For this review, take the finished solid that the model builds, in its own axes (mm). Face numbers are marked on the shaded views. A direction names the side the tool comes from. Coordinates: 2 decimals unless noted, no trailing zeros. Loops run counter-clockwise (first coordinate to the right, second up) from the corner with the lowest first, then second, coordinate; pieces in that order, holes last.
1. Take a section at C-C, the plane x = 1.2. State the section outline as (y, z) points, then the cut area to 3 significant figures.
2. Take a section at D-D, the plane z = 1.5. State the section outline as (x, y) points.
3. Clearance check with flat-ended pins moving along their axes: P1, Ø1, axis at x = 1.5, y = -0.5, coming from the +Z side; P2, Ø1, axis at x = -1, y = 4.5, coming from the +Z side; P3, Ø1, axis at y = 1.5, z = 1.5, coming from the -X side. State where each tip first meets the part, or that it passes through.
4. Take a section at A-A, the plane y = -0.5. State the section outline as (x, z) points (3 decimals), then the cut area to 3 significant figures.
5. Machinability: for the marked faces 1 and 2, which of the approach directions +Z, -Z, +X, -X, +Y, -Y give a long, thin tool a straight path to every point of the face, cutting with its end or side? Answer none if there is none.
6. To check wall thickness, follow probe 1 along Y at (x, z) = (0.4, -0.55); probe 2 along Z at (x, y) = (0.95, 4.5); probe 3 along Z at (x, y) = (1.35, 0.25). State the ranges of each line that lie inside material, in increasing order.
7. Take a section at B-B, the plane z = 0.1. State the section outline as (x, y) points (3 decimals).
8. Mouldability with a two-part tool opening along X and no side actions: class the marked faces 3, 4 and 5 as pulls with the +X half, pulls with the -X half, needs draft (parallel to the pull), parting line crosses it, or undercut.
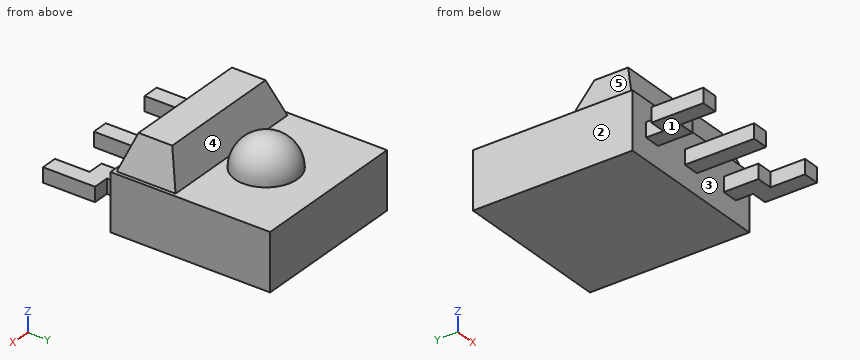
```python
from build123d import *

# Parameters (mm, degrees)
BOSS_EXTRUDE1_DEPTH   = 0.21
SKETCH1_W             = 0.47
SKETCH1_H             = 2
BOSS_EXTRUDE1_2_DEPTH = 0.21
BOSS_EXTRUDE1_3_DEPTH = 0.21
SKETCH2_W             = 4.6
SKETCH2_H             = 1.64
BOSS_EXTRUDE2_DEPTH   = 4.6
REVOLVE1_ANGLE        = 180
SKETCH4_W             = 4.4
SKETCH4_H             = 1.7
BOSS_EXTRUDE3_DEPTH   = 1
CHAMFER1_SIZE         = 1
CHAMFER1_SIZE_2       = 0.363970234


with BuildPart() as part:
    # Sketch1 → Boss-Extrude1 (new, symmetric)
    with BuildSketch(Plane.XY):
        Polygon((-1.295, 1), (-1.295, 0), (-1.765, 0), (-1.765, -1), (-2.235, -1), (-2.235, 0.5), (-1.765, 0.5), (-1.765, 1), align=None)
    extrude(amount=BOSS_EXTRUDE1_DEPTH, both=True)



with BuildPart() as body_2:
    # Sketch1 → Boss-Extrude1 2 (new, symmetric)
    with BuildSketch(Plane.XY):
        Rectangle(SKETCH1_W, SKETCH1_H)
    extrude(amount=BOSS_EXTRUDE1_2_DEPTH, both=True)


with BuildPart() as body_3:
    # Sketch1 → Boss-Extrude1 3 (new, symmetric)
    with BuildSketch(Plane.XY):
        Polygon((1.765, 1), (1.295, 1), (1.295, 0), (1.765, 0), (1.765, -1), (2.235, -1), (2.235, 0.5), (1.765, 0.5), align=None)
    extrude(amount=BOSS_EXTRUDE1_3_DEPTH, both=True)


with BuildPart() as part_1:
    add(part.part)

    add(body_2.part)  # Boss-Extrude2 merges body 2

    add(body_3.part)  # Boss-Extrude2 merges body 3
    # Sketch2 → Boss-Extrude2 (add)
    with BuildSketch(Plane(origin=(0, 1, 0), x_dir=(1, 0, 0), z_dir=(0, 1, 0))):
        Rectangle(SKETCH2_W, SKETCH2_H)
    extrude(amount=BOSS_EXTRUDE2_DEPTH)

    # Sketch3 → Revolve1 (revolve)
    with BuildSketch(Plane.XY.offset(0.82)):
        with BuildLine():
            Line((0, 4.7), (0, 2.9))
            ThreePointArc((0, 2.9), (0.9, 3.8), (0, 4.7))
        make_face()
    revolve(axis=Axis((0, 4.7, 0.82), (0, -1, 0)), revolution_arc=REVOLVE1_ANGLE)

    # Sketch4 → Boss-Extrude3 (add)
    with BuildSketch(Plane.XY.offset(0.82)):
        with Locations((0, 1.95)):
            Rectangle(SKETCH4_W, SKETCH4_H)
    extrude(amount=BOSS_EXTRUDE3_DEPTH)

    # Chamfer1
    # the kernel refuses this chamfer: 1, 0.363970234 mm, written as the material it takes off along each edge
    with BuildSketch(Plane(origin=(4.794194733, 1.1, 1.82), x_dir=(0, -0.013184058198646006, -0.9999130865277315), z_dir=(-1, 0, 0))) as chamfer1_piece_1_section:
        Polygon((CHAMFER1_SIZE * 0.999913086528, -CHAMFER1_SIZE * 0.0131840581986), (-CHAMFER1_SIZE_2 * 0.0131840582083, -CHAMFER1_SIZE_2 * 0.999913087259), (0, 0), align=None)
    chamfer1_piece_1 = extrude(amount=9.588389465, mode=Mode.PRIVATE)
    chamfer1_piece_1 = split(chamfer1_piece_1, bisect_by=Plane(origin=(0, 1.212526608, 0.82), z_dir=(0, 0, 1)), keep=Keep.TOP, mode=Mode.PRIVATE)
    add(chamfer1_piece_1, mode=Mode.SUBTRACT)
    with BuildSketch(Plane(origin=(-2.2, -1.494194733, 1.82), x_dir=(-0.013184058198646006, 0, -0.9999130865277315), z_dir=(0, 1, 0))) as chamfer1_piece_2_section:
        Polygon((CHAMFER1_SIZE * 0.999913086528, -CHAMFER1_SIZE * 0.0131840581986), (-CHAMFER1_SIZE_2 * 0.0131840582083, -CHAMFER1_SIZE_2 * 0.999913087259), (0, 0), align=None)
    chamfer1_piece_2 = extrude(amount=6.888389465, mode=Mode.PRIVATE)
    chamfer1_piece_2 = split(chamfer1_piece_2, bisect_by=Plane(origin=(-2.087473392, 1.95, 0.82), z_dir=(0, 0, 1)), keep=Keep.TOP, mode=Mode.PRIVATE)
    add(chamfer1_piece_2, mode=Mode.SUBTRACT)
    with BuildSketch(Plane(origin=(2.2, 5.394194733, 1.82), x_dir=(0.013184058198646006, 0, -0.9999130865277315), z_dir=(0, -1, 0))) as chamfer1_piece_3_section:
        Polygon((CHAMFER1_SIZE * 0.999913086528, -CHAMFER1_SIZE * 0.0131840581986), (-CHAMFER1_SIZE_2 * 0.0131840582083, -CHAMFER1_SIZE_2 * 0.999913087259), (0, 0), align=None)
    chamfer1_piece_3 = extrude(amount=6.888389465, mode=Mode.PRIVATE)
    chamfer1_piece_3 = split(chamfer1_piece_3, bisect_by=Plane(origin=(2.087473392, 1.95, 0.82), z_dir=(0, 0, 1)), keep=Keep.TOP, mode=Mode.PRIVATE)
    add(chamfer1_piece_3, mode=Mode.SUBTRACT)
    with BuildSketch(Plane(origin=(-4.794194733, 2.8, 1.82), x_dir=(0, 0.013184058198646006, -0.9999130865277315), z_dir=(1, 0, 0))) as chamfer1_piece_4_section:
        Polygon((CHAMFER1_SIZE * 0.999913086528, -CHAMFER1_SIZE * 0.0131840581986), (-CHAMFER1_SIZE_2 * 0.0131840582083, -CHAMFER1_SIZE_2 * 0.999913087259), (0, 0), align=None)
    chamfer1_piece_4 = extrude(amount=9.588389465, mode=Mode.PRIVATE)
    chamfer1_piece_4 = split(chamfer1_piece_4, bisect_by=Plane(origin=(0, 2.687473392, 0.82), z_dir=(0, 0, 1)), keep=Keep.TOP, mode=Mode.PRIVATE)
    add(chamfer1_piece_4, mode=Mode.SUBTRACT)


solid = part_1.part
```
Results list:
1. outline: (1, -0.82) - (5.6, -0.82) - (5.6, 0.82) - (2.8, 0.82) - (2.44, 1.82) - (1.46, 1.82) - (1.1, 0.82) - (1, 0.82) - close
1. area: 8.88 mm2
2. outline: (-1.95, 1.35) - (1.95, 1.35) - (1.95, 2.55) - (-1.95, 2.55) - close; circle Ø1.18 at (0, 3.8)
3. P1: stops at z = 0.21
3. P2: stops at z = 1.36
3. P3: stops at x = -2.13
4. outline: (-2.235, -0.21) - (-1.765, -0.21) - (-1.765, 0.21) - (-2.235, 0.21) - close; (-0.235, -0.21) - (0.235, -0.21) - (0.235, 0.21) - (-0.235, 0.21) - close; (1.765, -0.21) - (2.235, -0.21) - (2.235, 0.21) - (1.765, 0.21) - close
4. area: 0.592 mm2
5. face 1: -Z, +X, -X, -Y
5. face 2: +Z, -Z, -X, +Y, -Y
6. probe 1: y = 1 to 5.6
6. probe 2: z = -0.82 to 0.82
6. probe 3: z = -0.21 to 0.21
7. outline: (-2.3, 1) - (-1.765, 1) - (-1.765, 0.5) - (-2.235, 0.5) - (-2.235, -1) - (-1.765, -1) - (-1.765, 0) - (-1.295, 0) - (-1.295, 1) - (-0.235, 1) - (-0.235, -1) - (0.235, -1) - (0.235, 1) - (1.295, 1) - (1.295, 0) - (1.765, 0) - (1.765, -1) - (2.235, -1) - (2.235, 0.5) - (1.765, 0.5) - (1.765, 1) - (2.3, 1) - (2.3, 5.6) - (-2.3, 5.6) - close
8. face 3: undercut
8. face 4: needs draft
8. face 5: pulls with the -X half
